Input: part model. Units: mm. Frame: model coordinates. A direction names the side the tool comes from. Give positions to 0.01 mm unless a question says otherwise; leave off trailing zeros. Order: outer loops, then holes, each group sorted by start corner. A loop starts at its lowest first (then second) coordinate and runs counter-clockwise, first axis right, second up. Notation, with made-up numbers: M -19,23.5 L -2,23.5 A22 cw -2,45.5 Z; hole C 67,13.5 d1. An arc over 180 degrees is marked long. Use a Markdown table: item, result.
from build123d import *

# Parameters (mm, degrees)
SKETCH1_W           = 18
SKETCH1_H           = 12
SKETCH1_W_2         = 14
SKETCH1_H_2         = 8
BOSS_EXTRUDE1_DEPTH = 12
BOSS_EXTRUDE2_DEPTH = 18


with BuildPart() as part:
    # Sketch1 → Boss-Extrude1 (new body)
    with BuildSketch(Plane(origin=(0, 0, 0), x_dir=(1, 0, 0), z_dir=(0, 1, 0))):
        with Locations((9, 6)):
            Rectangle(SKETCH1_W, SKETCH1_H)
        with Locations((9, 6)):
            Rectangle(SKETCH1_W_2, SKETCH1_H_2, mode=Mode.SUBTRACT)
    extrude(amount=BOSS_EXTRUDE1_DEPTH)

    # Sketch2 → Boss-Extrude2 (add)
    with BuildSketch(Plane(origin=(18, 0, 0), x_dir=(0, 0, -1), z_dir=(1, 0, 0))):
        Polygon((6, 17), (0, 12), (12, 12), align=None)
    extrude(amount=-BOSS_EXTRUDE2_DEPTH)


solid = part.part
1) Mould query, pull axis X, two halves, no side actions, for faces 3 (the face through (9, 6, -12)), 4 (the face through (18, 7, -6)), 5 (the face through (16, 6, -6)). Classes: released by +X, released by -X, zero draft, split by the parting line, or undercut.
Response values:
| item | result |
|---|---|
| face 3 | zero draft |
| face 4 | released by +X |
| face 5 | undercut |
2) Cut plane D-D on y = 15.75. Return loops of the section in (x, z), and give its area (3 significant figures).
Response values:
| item | result |
|---|---|
| outline | M 0,-7.5 L 18,-7.5 L 18,-4.5 L 0,-4.5 Z |
| area | 54.0 mm² |
3) Cut plane B-B on x = 2.75. Return loops of the section in (y, z), and give its area (3 significant figures).
Response values:
| item | result |
|---|---|
| outline | M 0,-12 L 12,-12 L 17,-6 L 12,0 L 0,0 L 0,-2 L 12,-2 L 12,-10 L 0,-10 Z |
| area | 78.0 mm² |
4) Cut plane C-C on z = -3. Return loops of the section in (x, y).
Response values:
| item | result |
|---|---|
| outline | M 0,0 L 2,0 L 2,12 L 16,12 L 16,0 L 18,0 L 18,14.5 L 0,14.5 Z |
5) First-contact query: pin 1 Ø2.5 at (y, z) = (8.5, -4.5) entering from -X. Flat tip, straight axial feed; report the tip coordinate or a pass-through.
Response values:
| item | result |
|---|---|
| pin 1 | stops at x = 0 |
6) Reachability of faces 1 (the face through (9.1, 14.5, -9)), 2 (the face through (9, 6, -2)) from +Z, -Z, +X, -X, +Y, -Y: full face, straight path, thin tool, end or side. Return the list, or none.
Response values:
| item | result |
|---|---|
| face 1 | -Z, +X, -X, +Y |
| face 2 | -Y |
7) Material intervals for line 1 (X direction, y = 11.75, z = -8.75); line 2 (Z direction, x = 4, y = 11.25); line 3 (Y direction, x = 1.75, z = -3.75) (3 decimals), sorted ascending. Write a range as from..to.
Response values:
| item | result |
|---|---|
| line 1 | x = 0..2, 16..18 |
| line 2 | z = -12..-10, -2..0 |
| line 3 | y = 0..15.125 |
8) Cut plane A-A on y = 7.25. Return loops of the section in (x, z), and give its area (3 significant figures).
Response values:
| item | result |
|---|---|
| outline | M 0,-12 L 18,-12 L 18,0 L 0,0 Z; hole M 2,-10 L 16,-10 L 16,-2 L 2,-2 Z |
| area | 104 mm² |
